from build123d import *

# Parameters (mm, degrees)
DODANIE_WYCI_GNI_CIE1_DEPTH      = 10
DODANIE_WYCI_GNI_CIE2_DEPTH      = 8
DODANIE_WYCI_GNI_CIE2_DEPTH_BACK = 46
SZKIC2_R                         = 17.5
DODANIE_WYCI_GNI_CIE3_DEPTH      = 4
DODANIE_WYCI_GNI_CIE3_DEPTH_BACK = 42
SZKIC3_R                         = 17.5
WYTNIJ_WYCI_GNI_CIE1_REACH       = 438.69
SZKIC4_R                         = 11.5
WYTNIJ_WYCI_GNI_CIE2_REACH       = 438.213
SZKIC5_R                         = 11.5
ZAOKR_GLENIE1_R                  = 4
ZAOKR_GLENIE2_R                  = 10
SZKIC7_R                         = 6.5
WYTNIJ_WYCI_GNI_CIE3_DEPTH       = 436.773035366


with BuildPart() as part:
    # Szkic1 → Dodanie-wyci_gni_cie1 (new body)
    with BuildSketch(Plane(origin=(0, 0, 0), x_dir=(0, 0, -1), z_dir=(1, 0, 0))):
        Polygon((0, 0), (271, 0), (407.197713576, -75.495625423), (408.756953924, -80.933342732), (393.243046076, -108.921173361), (387.805328767, -110.480413708), (260.655296626, -40), (0, -40), (-4, -36), (-4, -4), align=None)
    extrude(amount=DODANIE_WYCI_GNI_CIE1_DEPTH)


with BuildPart() as body_2:
    # Lustro3: mirrored copy
    add(part.part.mirror(Plane.ZY.offset(9)))


with BuildPart() as part_1:
    add(part.part)

    add(body_2.part)  # Dodanie-wyci_gni_cie2 merges body 2
    # Szkic2 → Dodanie-wyci_gni_cie2 (add, two sides: drawn at the far end of the back side and taken through both)
    with BuildSketch(Plane(origin=(10, 0, 0), x_dir=(0, 0, -1), z_dir=(1, 0, 0)).offset(-DODANIE_WYCI_GNI_CIE2_DEPTH_BACK)):
        with Locations((-4, -20)):
            Circle(SZKIC2_R)
    extrude(amount=DODANIE_WYCI_GNI_CIE2_DEPTH + DODANIE_WYCI_GNI_CIE2_DEPTH_BACK)

    # Szkic3 → Dodanie-wyci_gni_cie3 (add, two sides: drawn at the far end of the back side and taken through both)
    with BuildSketch(Plane(origin=(10, 0, 0), x_dir=(0, 0, -1), z_dir=(1, 0, 0)).offset(-DODANIE_WYCI_GNI_CIE3_DEPTH_BACK)):
        with Locations((401, -94.927258046)):
            Circle(SZKIC3_R)
    extrude(amount=DODANIE_WYCI_GNI_CIE3_DEPTH + DODANIE_WYCI_GNI_CIE3_DEPTH_BACK)

    # Szkic4 → Wytnij-wyci_gni_cie1 (cut, up to next)
    with BuildSketch(Plane(origin=(18, 0, 0), x_dir=(0, 0, -1), z_dir=(1, 0, 0)), mode=Mode.PRIVATE) as wytnij_wyci_gni_cie1_sk1:
        with Locations((-4, -20)):
            Circle(SZKIC4_R)
    wytnij_wyci_gni_cie1_tool1 = extrude(wytnij_wyci_gni_cie1_sk1.sketch, amount=-WYTNIJ_WYCI_GNI_CIE1_REACH, mode=Mode.PRIVATE) & part_1.part
    add(wytnij_wyci_gni_cie1_tool1.solids().sort_by_distance((18, -20, 4))[0], mode=Mode.SUBTRACT)

    # Szkic5 → Wytnij-wyci_gni_cie2 (cut, up to next)
    with BuildSketch(Plane(origin=(14, 0, 0), x_dir=(0, 0, -1), z_dir=(1, 0, 0)), mode=Mode.PRIVATE) as wytnij_wyci_gni_cie2_sk1:
        with Locations((401, -94.927258046)):
            Circle(SZKIC5_R)
    wytnij_wyci_gni_cie2_tool1 = extrude(wytnij_wyci_gni_cie2_sk1.sketch, amount=-WYTNIJ_WYCI_GNI_CIE2_REACH, mode=Mode.PRIVATE) & part_1.part
    add(wytnij_wyci_gni_cie2_tool1.solids().sort_by_distance((14, -94.927258, -401))[0], mode=Mode.SUBTRACT)

    # Zaokr_glenie1
    # the kernel refuses this fillet: 4 mm, written as the material it adds along each edge
    with BuildSketch(Plane(origin=(-28, -94.927258046, -401), x_dir=(0, 0.5436759874947165, -0.8392951927788249), z_dir=(0, -0.8392951927788249, -0.5436759874947165))) as zaokr_glenie1_piece_1_section:
        with BuildLine():
            CenterArc((17.5 + ZAOKR_GLENIE1_R, -ZAOKR_GLENIE1_R), ZAOKR_GLENIE1_R, 90, 90)
            Line((17.5 + ZAOKR_GLENIE1_R, 0), (17.5, 0))
            Line((17.5, 0), (17.5, -ZAOKR_GLENIE1_R))
        make_face()
    zaokr_glenie1_piece_1 = revolve(axis=Axis((-28, -94.927258046, -401), (1, 0, 0)), revolution_arc=236.131536778, mode=Mode.PRIVATE)
    zaokr_glenie1_piece_1 = split(zaokr_glenie1_piece_1, bisect_by=Plane(origin=(-29.129078487, -79.146319532, -408.244533267), z_dir=(0, -0.27563735581700194, 0.9612616959383181)), keep=Keep.TOP, mode=Mode.PRIVATE)
    zaokr_glenie1_piece_1 = split(zaokr_glenie1_piece_1, bisect_by=Plane(origin=(-29.129078487, -109.433594017, -391.456022876), z_dir=(0, 0.961261695938321, 0.2756373558169916)), keep=Keep.TOP, mode=Mode.PRIVATE)
    zaokr_glenie1_piece_1 = split(zaokr_glenie1_piece_1, bisect_by=Plane(origin=(-29.129078487, -103.388095722, -375.010448424), z_dir=(0, 0.8746197071393952, -0.4848096202463382)), keep=Keep.TOP, mode=Mode.PRIVATE)
    zaokr_glenie1_piece_1 = split(zaokr_glenie1_piece_1, bisect_by=Plane(origin=(-29.129078487, -68.403307437, -394.402833234), z_dir=(0, -0.8746197071393943, 0.4848096202463399)), keep=Keep.TOP, mode=Mode.PRIVATE)
    add(zaokr_glenie1_piece_1)
    with BuildSketch(Plane(origin=(-28, -20, 4), x_dir=(0, -0.8826991233352643, 0.469938567967299), z_dir=(0, 0.469938567967299, 0.8826991233352643))) as zaokr_glenie1_piece_2_section:
        with BuildLine():
            CenterArc((17.5 + ZAOKR_GLENIE1_R, -ZAOKR_GLENIE1_R), ZAOKR_GLENIE1_R, 90, 90)
            Line((17.5 + ZAOKR_GLENIE1_R, 0), (17.5, 0))
            Line((17.5, 0), (17.5, -ZAOKR_GLENIE1_R))
        make_face()
    zaokr_glenie1_piece_2 = revolve(axis=Axis((-28, -20, 4), (1, 0, 0)), revolution_arc=118.030308923, mode=Mode.PRIVATE)
    zaokr_glenie1_piece_2 = split(zaokr_glenie1_piece_2, bisect_by=Plane(origin=(-29.137845044, -41.167759306, -1.167759306), z_dir=(0, 0.7071067811865419, -0.7071067811865531)), keep=Keep.TOP, mode=Mode.PRIVATE)
    zaokr_glenie1_piece_2 = split(zaokr_glenie1_piece_2, bisect_by=Plane(origin=(-29.137845044, -40, -9.710667039), z_dir=(0, 1, 0)), keep=Keep.TOP, mode=Mode.PRIVATE)
    add(zaokr_glenie1_piece_2)
    with BuildSketch(Plane(origin=(10, -20, 4), x_dir=(0, -0.8826991233352602, 0.46993856796730693), z_dir=(0, 0.46993856796730693, 0.8826991233352602))) as zaokr_glenie1_piece_3_section:
        with BuildLine():
            CenterArc((17.5 + ZAOKR_GLENIE1_R, ZAOKR_GLENIE1_R), ZAOKR_GLENIE1_R, 180, 90)
            Line((17.5, ZAOKR_GLENIE1_R), (17.5, 0))
            Line((17.5, 0), (17.5 + ZAOKR_GLENIE1_R, 0))
        make_face()
    zaokr_glenie1_piece_3 = revolve(axis=Axis((10, -20, 4), (1, 0, 0)), revolution_arc=118.030308923, mode=Mode.PRIVATE)
    zaokr_glenie1_piece_3 = split(zaokr_glenie1_piece_3, bisect_by=Plane(origin=(11.137845044, -41.167759305, -1.167759305), z_dir=(0, 0.7071067811865419, -0.7071067811865531)), keep=Keep.TOP, mode=Mode.PRIVATE)
    zaokr_glenie1_piece_3 = split(zaokr_glenie1_piece_3, bisect_by=Plane(origin=(11.137845044, -40, -9.710667039), z_dir=(0, 1, 0)), keep=Keep.TOP, mode=Mode.PRIVATE)
    add(zaokr_glenie1_piece_3)
    with BuildSketch(Plane(origin=(10, -94.927258046, -401), x_dir=(0, 0.5436759874947362, -0.8392951927788123), z_dir=(0, -0.8392951927788123, -0.5436759874947362))) as zaokr_glenie1_piece_4_section:
        with BuildLine():
            CenterArc((17.5 + ZAOKR_GLENIE1_R, ZAOKR_GLENIE1_R), ZAOKR_GLENIE1_R, 180, 90)
            Line((17.5, ZAOKR_GLENIE1_R), (17.5, 0))
            Line((17.5, 0), (17.5 + ZAOKR_GLENIE1_R, 0))
        make_face()
    zaokr_glenie1_piece_4 = revolve(axis=Axis((10, -94.927258046, -401), (1, 0, 0)), revolution_arc=236.131536778, mode=Mode.PRIVATE)
    zaokr_glenie1_piece_4 = split(zaokr_glenie1_piece_4, bisect_by=Plane(origin=(11.12907849, -68.403307435, -394.402833232), z_dir=(0, -0.8746197071393943, 0.4848096202463399)), keep=Keep.TOP, mode=Mode.PRIVATE)
    zaokr_glenie1_piece_4 = split(zaokr_glenie1_piece_4, bisect_by=Plane(origin=(11.12907849, -103.388095721, -375.010448422), z_dir=(0, 0.8746197071393952, -0.4848096202463382)), keep=Keep.TOP, mode=Mode.PRIVATE)
    zaokr_glenie1_piece_4 = split(zaokr_glenie1_piece_4, bisect_by=Plane(origin=(11.12907849, -109.433594018, -391.456022874), z_dir=(0, 0.961261695938321, 0.2756373558169916)), keep=Keep.TOP, mode=Mode.PRIVATE)
    zaokr_glenie1_piece_4 = split(zaokr_glenie1_piece_4, bisect_by=Plane(origin=(11.12907849, -79.14631953, -408.244533267), z_dir=(0, -0.27563735581700194, 0.9612616959383181)), keep=Keep.TOP, mode=Mode.PRIVATE)
    add(zaokr_glenie1_piece_4)
    with BuildSketch(Plane(origin=(10, -20, 4), x_dir=(0, 0, -1), z_dir=(0, -1, 0))) as zaokr_glenie1_piece_5_section:
        with BuildLine():
            CenterArc((17.5 + ZAOKR_GLENIE1_R, ZAOKR_GLENIE1_R), ZAOKR_GLENIE1_R, 180, 90)
            Line((17.5, ZAOKR_GLENIE1_R), (17.5, 0))
            Line((17.5, 0), (17.5 + ZAOKR_GLENIE1_R, 0))
        make_face()
    zaokr_glenie1_piece_5 = revolve(axis=Axis((10, -20, 4), (1, 0, 0)), revolution_arc=118.030308923, mode=Mode.PRIVATE)
    zaokr_glenie1_piece_5 = split(zaokr_glenie1_piece_5, bisect_by=Plane(origin=(11.137845049, 0, -9.710667043), z_dir=(0, -1, 0)), keep=Keep.TOP, mode=Mode.PRIVATE)
    zaokr_glenie1_piece_5 = split(zaokr_glenie1_piece_5, bisect_by=Plane(origin=(11.137845049, 1.167759309, -1.167759309), z_dir=(0, -0.7071067811865533, -0.7071067811865418)), keep=Keep.TOP, mode=Mode.PRIVATE)
    add(zaokr_glenie1_piece_5)
    with BuildSketch(Plane(origin=(-28, -20, 4), x_dir=(0, 0, -1), z_dir=(0, -1, 0))) as zaokr_glenie1_piece_6_section:
        with BuildLine():
            CenterArc((17.5 + ZAOKR_GLENIE1_R, -ZAOKR_GLENIE1_R), ZAOKR_GLENIE1_R, 90, 90)
            Line((17.5 + ZAOKR_GLENIE1_R, 0), (17.5, 0))
            Line((17.5, 0), (17.5, -ZAOKR_GLENIE1_R))
        make_face()
    zaokr_glenie1_piece_6 = revolve(axis=Axis((-28, -20, 4), (1, 0, 0)), revolution_arc=118.030308923, mode=Mode.PRIVATE)
    zaokr_glenie1_piece_6 = split(zaokr_glenie1_piece_6, bisect_by=Plane(origin=(-29.137845048, 1.167759309, -1.167759309), z_dir=(0, -0.7071067811865533, -0.7071067811865418)), keep=Keep.TOP, mode=Mode.PRIVATE)
    zaokr_glenie1_piece_6 = split(zaokr_glenie1_piece_6, bisect_by=Plane(origin=(-29.137845048, 0, -9.710667042), z_dir=(0, -1, 0)), keep=Keep.TOP, mode=Mode.PRIVATE)
    add(zaokr_glenie1_piece_6)

    # Zaokr_glenie2
    zaokr_glenie2_edges = [part_1.edges().sort_by_distance(p)[0] for p in [
        (5, 0, -271),
        (5, -40, -260.655296626),
        (-23, -40, -260.655296626),
        (-23, 0, -271),
    ]]
    fillet(zaokr_glenie2_edges, radius=ZAOKR_GLENIE2_R)

    # Szkic7 → Wytnij-wyci_gni_cie3 (cut, through all)
    with BuildSketch(Plane(origin=(10, 0, 0), x_dir=(0, 0, -1), z_dir=(1, 0, 0))):
        with Locations(Location((351, -67.211805474, 0), (0, 0, 180))):
            Circle(SZKIC7_R)
    extrude(amount=-WYTNIJ_WYCI_GNI_CIE3_DEPTH, mode=Mode.SUBTRACT)


solid = part_1.part
Check sheet for the modelled part. Datum: model origin and axes. Units: mm. A direction names the side the tool comes from. Give positions to 0.01 mm unless a question says otherwise; leave off trailing zeros. Loops run counter-clockwise (first coordinate to the right, second up) from the corner with the lowest first, then second, coordinate; pieces in that order, holes last. Notation, with made-up numbers: M -24.75,76.5 L -18.75,76.5 A22 ccw -18.75,83.5 Z; hole C 74,26.5 d5. An arc over 180 degrees is marked long. Answer as a JSON object with one key per item and string values. Group by question number.
Q1. Material ranges on line 1 along X through (y, z) = (-30, -266.5); line 2 along X through (y, z) = (-35.5, -9.5); line 3 along Y through (x, z) = (-22, 4), recorded low to high. Write a range as [from, to].
Q2. Cross-section at B-B on x = -22. Record the cut outline in (y, z).
Q3. Go/stop test with flat-tipped pins: P1, Ø11, axis at x = -21, z = -143.5, coming from the -Y side; P2, Ø1.5, axis at x = 1, z = -219.5, coming from the +Y side; P3, Ø1, axis at x = -16, y = -88, coming from the +Z side; P4, Ø15, axis at y = -67.21, z = -351, coming from the +X side. Record where each tip stops, or that it passes through.
Q4. Access from +Z, -Z, +X, -X, +Y, -Y to the whole of each face (thin tool, end or side, straight path). Record for faces 1 (the flat face through (5, -40, -131)), 2 (the flat face through (-32, -99, -412)), 3 (the cylindrical face through (-9.378, -19.231, 21.483)).
Q5. Release check for a two-part mould opening along X. For faces 4 (the cylindrical face through (-22.93, -69.16, -344.8)), 5 (the flat face through (-18, -26, -204)), 6 (the flat face through (14, -99, -412)) record: released by +X, released by -X, zero draft, split by the parting line, or undercut.
Q6. Cross-section at D-D on x = -4. Record the cut outline in (y, z).
Q7. Cross-section at A-A on z = -114. Record the cut outline in (x, y), then the cut area to 3 significant figures.
Q8. Cross-section at C-C on z = -351. Record the cut outline in (x, y).
Evaluation:
{
 "1": {"line 1": "x = [-28, -18], [0, 10]", "line 2": "x = [-28.11, -18], [0, 10.11]", "line 3": "y = [-37.5, -31.5], [-8.5, -2.5]"},
 "2": {"outline": "M -110.48,-387.81 L -109.48,-391.28 A17.5 ccw long -78.97,-408.2 L -75.5,-407.2 L -1.25,-273.26 A10 ccw 0,-268.41 L 0,0 L -2.56,2.56 A17.5 ccw long -37.44,2.56 L -40,0 L -40,-258.07 A10 cw -41.25,-262.92 Z; hole C -94.93,-401 d23; hole C -67.21,-351 d13; hole C -20,4 d23"},
 "3": {"P1": "stops at y = -40", "P2": "stops at y = 0", "P3": "stops at z = -384.72", "P4": "stops at x = 10"},
 "4": {"face 1": "+Z, +X, -X, -Y", "face 2": "+Z, -Z, -X, +Y, -Y", "face 3": "none"},
 "5": {"face 4": "zero draft", "face 5": "undercut", "face 6": "released by +X"},
 "6": {"outline": "C -94.93,-401 d35; C -20,4 d35; hole C -94.93,-401 d23; hole C -20,4 d23"},
 "7": {"outline": "M -28,-40 L -18,-40 L -18,0 L -28,0 Z; M 0,-40 L 10,-40 L 10,0 L 0,0 Z", "area": "800 mm2"},
 "8": {"outline": "M -28,-90.08 L -18,-90.08 L -18,-73.71 L -28,-73.71 Z; M -28,-60.71 L -18,-60.71 L -18,-44.34 L -28,-44.34 Z; M 0,-90.08 L 10,-90.08 L 10,-73.71 L 0,-73.71 Z; M 0,-60.71 L 10,-60.71 L 10,-44.34 L 0,-44.34 Z"}
}
